Read the model definition and answer for the solid it produces. Units are mm, in the model's axes. Face numbers are marked on the shaded views. A direction names the side the tool comes from. Give positions to 0.01 mm unless a question says otherwise; leave off trailing zeros. Write each loop counter-clockwise with the first axis right and the second up, starting at its lowest first coordinate (ties: lowest second). Pieces come first, ordered by that corner, then holes. Notation, with made-up numbers: (3.25, 11.5) -> (9.25, 11.5) arc R18 ccw to (9.25, 15.5) -> close; hole circle Ø11 at (11.5, 48.5). An arc over 180 degrees is marked (long way). Use a Markdown table: item, result.
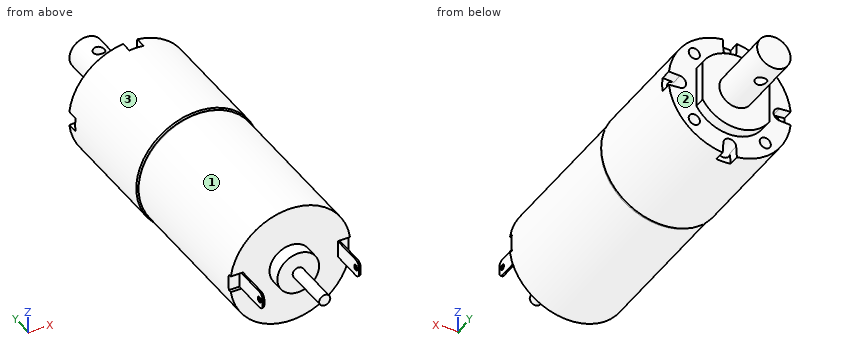
Autodesk Fusion 360 part; units mm, degrees
sketch "Sketch1" plane through (0, 0, 0) normal (0, 1, 0) x (1, 0, 0)
  circle A0 centre (0, 0) radius 11
  circle A1 centre (0, 0) radius 10.8
  dimension "d1" = 22
  dimension "d4" = 21.6
extrude "Extrude1" add sketch "Sketch1" along normal blind 21.4 contours A0 | A1 makes body 1
extrude "Extrude2" add sketch "Sketch1" against normal blind 29.5 separate body contours A1 makes body 2
sketch "Sketch2" plane through (0, -29.5, 0) normal (0, -1, 0) x (1, 0, 0)
  circle A0 centre (0, 0) radius 10.8
  circle A1 centre (0, 0) radius 3.75
  circle A2 centre (0, 0) radius 1
  dimension "d7" = 7.5
  dimension "d8" = 2
extrude "Extrude3" add sketch "Sketch2" along normal blind 2.5 contours A1 | A2 bodies 2
sketch "Sketch3" plane through (0, -29.5, 0) normal (0, -1, 0) x (1, 0, 0)
  circle A0 centre (0, 0) radius 3.75
  circle A1 centre (0, 0) radius 10.8
  line L0 (0, 0) -> (10.8, 0) construction
  line L1 (0, 0) -> (0, 10.8) construction
  line L2 (8.5, -1.5) -> (8.8, -1.5)
  line L3 (8.8, -1.5) -> (8.8, 1.5)
  line L4 (8.8, 1.5) -> (8.5, 1.5)
  line L5 (8.5, 1.5) -> (8.5, -1.5)
  line L6 (8.5, -1.5) -> (8.8, 1.5) construction
  line L7 (8.8, -1.5) -> (8.5, 1.5) construction
  line L8 (-8.8, -1.5) -> (-8.5, 1.5) construction
  line L9 (-8.5, 1.5) -> (-8.5, -1.5)
  line L10 (-8.8, -1.5) -> (-8.8, 1.5)
  line L11 (0, 0) -> (-10.8, 0) construction
  line L12 (-8.5, -1.5) -> (-8.8, 1.5) construction
  line L13 (-8.8, 1.5) -> (-8.5, 1.5)
  line L14 (-8.5, -1.5) -> (-8.8, -1.5)
  line L15 (-8.8, 1.5) -> (-10.6953, 1.5)
  line L16 (-8.8, -1.5) -> (-10.6953, -1.5)
  circle A2 centre (0, 0) radius 10.8
  line L17 (8.8, 1.5) -> (10.6953, 1.5)
  line L18 (8.8, -1.5) -> (10.6953, -1.5)
  point P0 (8.65, 0)
  dimension "d14" = 0.3
  dimension "d15" = 3
  dimension "d16" = 2
extrude "Extrude5" add sketch "Sketch3" along normal blind 6.75 contours L2 L3 L4 L5 | L9 L10 L13 L14 bodies 2
sketch "Sketch4" plane through (-8.8, 0, 0) normal (-1, 0, 0) x (0, 0, 1)
  line L0 (1.5, -29.5) -> (-1.5, -29.5)
  line L1 (-1.5, -29.5) -> (-1.5, -36.25)
  line L2 (-1.5, -36.25) -> (1.5, -36.25)
  line L3 (1.5, -36.25) -> (1.5, -29.5)
  circle A0 centre (0, -35.25) radius 0.5
  dimension "d19" = 1
  dimension "d20" = 1
  dimension "d21" = 1.5
extrude "Extrude6" cut sketch "Sketch4" against normal blind 1000 contours A0 bodies 2
fillet "Fillet1" radius 1 4 edges at (-8.65, -36.25, -1.5) (-8.65, -36.25, 1.5) (8.65, -36.25, 1.5) (8.65, -36.25, -1.5) on bodies 2
extrude "Extrude7" add sketch "Sketch2" along normal blind 8.4 from surface at 2.5 separate body contours A2 makes body 3
sketch "Sketch5" plane through (0, 21.4, 0) normal (0, 1, 0) x (-1, 0, 0)
  circle A0 centre (0, 0) radius 11
  line L0 (6, -3.625) -> (-6, -3.625)
  line L1 (-6, -3.625) -> (-6, 3.625)
  line L2 (-6, 3.625) -> (6, 3.625)
  line L3 (6, 3.625) -> (6, -3.625)
  line L4 (6, -3.625) -> (-6, 3.625) construction
  line L5 (-6, -3.625) -> (6, 3.625) construction
  line L6 (6, -3.625) -> (6, 3.625)
  arc A1 (-6, -3.6056) -> (6, -3.6056) centre (0, 0) ccw
  arc A2 (6, 3.6056) -> (-6, 3.6056) centre (0, 0) ccw
  circle A3 centre (0, 0) radius 3
  circle A4 centre (0, 0) radius 9
  line L7 (0, 0) -> (0, -11) construction
  line L8 (0, 0) -> (0, 11) construction
  line L9 (0, 0) -> (-11, 0) construction
  line L10 (0, 0) -> (11, 0) construction
  circle A5 centre (9, 0) radius 1.15
  circle A6 centre (0, 9) radius 1.15
  circle A7 centre (-9, 0) radius 1.15
  circle A8 centre (0, -9) radius 1.15
  line L11 (8.9265, -1.1477) -> (10.9258, -1.2756)
  line L12 (8.9265, 1.1477) -> (10.9258, 1.2756)
  line L13 (-8.9265, -1.1477) -> (-10.9258, -1.2756)
  line L14 (-8.9265, 1.1477) -> (-10.9258, 1.2756)
  line L15 (-1.1477, -8.9265) -> (-1.2756, -10.9258)
  line L16 (1.1477, -8.9265) -> (1.2756, -10.9258)
  line L17 (1.1477, 8.9265) -> (1.2756, 10.9258)
  line L18 (-1.1477, 8.9265) -> (-1.2756, 10.9258)
  line L19 (0, 0) -> (-6.3679, 6.36) construction
  circle A9 centre (-6.3679, 6.36) radius 1
  circle A10 centre (6.3679, 6.36) radius 1
  circle A11 centre (-6.3679, -6.36) radius 1
  circle A12 centre (6.3679, -6.36) radius 1
  dimension "d32" = 14
  dimension "d33" = 12
  dimension "d34" = 7.25
  dimension "d37" = 6
  dimension "d40" = 18
  dimension "d41" = 2.3
  dimension "d42" = 2.3
  dimension "d43" = 2.3
  dimension "d44" = 2.3
  dimension "d49" = 2
extrude "Extrude8" add sketch "Sketch5" along normal blind 2 contours L0 A1 | L0 L1 L2 L3 L6 A1 A2 | L2 A2 | A3 bodies 1
extrude "Extrude9" add sketch "Sketch5" along normal blind 14 contours A3 bodies 1
extrude "Extrude10" cut sketch "Sketch5" against normal blind 2 contours A0 A5 L11 L12 | A0 A6 L17 L18 | A4 A5 | A4 A5 | A0 A8 L15 L16 | A4 A6 | A4 A6 | A4 A8 | A4 A8 | A0 A7 L13 L14 | A4 A7 | A4 A7 bodies 1
extrude "Extrude11" cut sketch "Sketch5" against normal blind 6.5 contours A4 A5 | A4 A5 | A4 A6 | A4 A6 | A4 A8 | A4 A8 | A4 A7 | A4 A7 bodies 1
extrude "Extrude12" cut sketch "Sketch5" against normal blind 4 contours A4 A10 | A4 A10 | A4 A12 | A4 A12 | A4 A9 | A4 A9 | A4 A11 | A4 A11 bodies 1
ref_plane "WorkPlane1" through (0, 31.7967, 3) normal (0, 0, 1) x (-1, 0, 0)
sketch "Sketch6" plane through (0, 0, 3) normal (0, 0, 1) x (1, 0, 0)
  line L0 (3, 35.4) -> (-3, 35.4)
  line L1 (-3, 23.4) -> (3, 23.4)
  circle A0 centre (0, 31.3) radius 1
  dimension "d53" = 2
  dimension "d54" = 4.1
extrude "Extrude13" cut sketch "Sketch6" against normal blind 99 bodies 1
fillet "Fillet2" radius 0.5 1 edges at (-10.0691, 0, 3.9054) on bodies 2
extrude "Extrude14" cut sketch "Sketch3" against normal blind 0.6 contours A1 L3 A2 L17 L18 | A1 L10 L15 L16 A2 bodies 2
combine "Combine1" operation add target body 2 tool bodies 3
combine "Combine2" operation add target body 1 tool bodies 2
Item 1: A cutting plane is placed at B-B (y = -1.5). Give the vertices of the cut face in (x, z), then the cut area to 3 significant figures.
Return value:
| item | result |
|---|---|
| outline | circle Ø21.6 at (0, 0) |
| area | 366 mm^2 |
Item 2: A cutting plane is placed at A-A (y = -33). Give the vertices of the cut face in (x, z), then the cut area to 3 significant figures.
Return value:
| item | result |
|---|---|
| outline | (-8.8, -1.5) -> (-8.5, -1.5) -> (-8.5, 1.5) -> (-8.8, 1.5) -> close; circle Ø2 at (0, 0); (8.5, -1.5) -> (8.8, -1.5) -> (8.8, 1.5) -> (8.5, 1.5) -> close |
| area | 4.94 mm^2 |
Item 3: A cutting plane is placed at C-C (y = 31.3). Give the vertices of the cut face in (x, z).
Return value:
| item | result |
|---|---|
| outline | (-1, -2.83) -> (-1, 2.83) arc R3 ccw to start; (1, -2.83) arc R3 ccw to (1, 2.83) -> close |
Item 4: Each of these flat-tipped pins is pushed along its axis until it touches: P1, Ø1.5, axis at x = -5, y = 6, coming from the +Z side; P2, Ø1.7, axis at x = -0.5, z = 10, coming from the +Y side; P3, Ø3, axis at x = -7.5, y = -28.5, coming from the +Z side; P4, Ø1, axis at y = 25, z = -5, coming from the -X side. Where does it stop, or does it pass through?
Return value:
| item | result |
|---|---|
| P1 | z = 10.15 |
| P2 | y = 21.4 |
| P3 | z = 8.98 |
| P4 | through |
Item 5: A tool of negligible diameter and unlimited length cuts with its end or side. For the marked faces 1, 2 and 3, from which of +Z, -Z, +X, -X, +Y, -Y can it reach the whole face along a straight path? Write none if from no direction.
Return value:
| item | result |
|---|---|
| face 1 | -Y |
| face 2 | +Y |
| face 3 | +Y, -Y |
Item 6: Straight lines are drawn through the part: line 1 along X through (y, z) = (19.25, 0); line 2 along Y through (x, z) = (8.7, 0). For each, find the intervals that lie inside material, in ascending order. Write a range as [from, to].
Return value:
| item | result |
|---|---|
| line 1 | [-11, -10.15], [-7.85, 7.85], [10.15, 11] |
| line 2 | [-36.25, -35.75], [-34.75, 14.9] |
